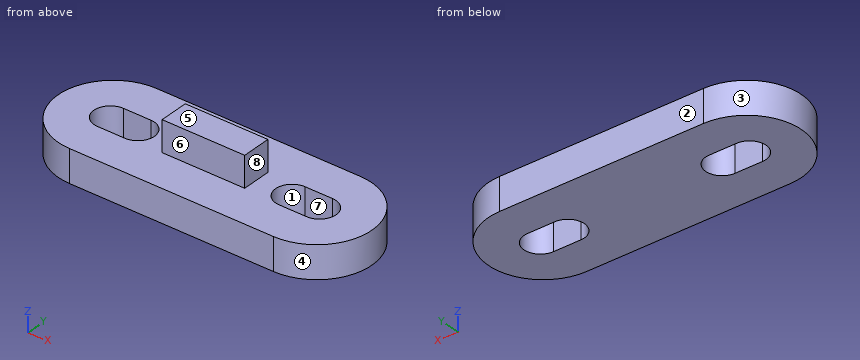
from build123d import *

# Parameters (mm, degrees)
BOSS_EXTRUDE2_DEPTH = 2.97
SKETCH5_W           = 7.5
SKETCH5_H           = 2.65
BOSS_EXTRUDE3_DEPTH = 2.8


with BuildPart() as part:
    # Sketch3 → Boss-Extrude2 (new body)
    with BuildSketch(Plane.XY):
        with BuildLine():
            Line((-9.25, 5), (9.25, 5))
            ThreePointArc((9.25, 5), (14.25, 0), (9.25, -5))
            Line((9.25, -5), (-9.25, -5))
            ThreePointArc((-9.25, -5), (-14.25, 0), (-9.25, 5))
        make_face()
        with BuildLine():
            Line((-9.5, 1.5), (-7, 1.5))
            ThreePointArc((-7, 1.5), (-5.5, 0), (-7, -1.5))
            Line((-7, -1.5), (-9.5, -1.5))
            ThreePointArc((-9.5, -1.5), (-11, 0), (-9.5, 1.5))
        make_face(mode=Mode.SUBTRACT)
        with BuildLine():
            Line((9.5, -1.5), (7, -1.5))
            ThreePointArc((7, -1.5), (5.5, 0), (7, 1.5))
            Line((7, 1.5), (9.5, 1.5))
            ThreePointArc((9.5, 1.5), (11, 0), (9.5, -1.5))
        make_face(mode=Mode.SUBTRACT)
    extrude(amount=BOSS_EXTRUDE2_DEPTH)

    # Sketch5 → Boss-Extrude3 (add)
    with BuildSketch(Plane.XY.offset(2.97)):
        Rectangle(SKETCH5_W, SKETCH5_H)
    extrude(amount=BOSS_EXTRUDE3_DEPTH)


solid = part.part
Check sheet for the modelled part. Datum: model origin and axes. Units: mm. Face numbers are marked on the shaded views. A direction names the side the tool comes from. Round coordinates to 2 decimals unless told otherwise and drop trailing zeros. Order: outer loops, then holes, each group sorted by start corner. A loop starts at its lowest first (then second) coordinate and runs counter-clockwise, first axis right, second up.
Q1. Draft check along Y on the marked faces 1, 2 and 3. Enter one of: pulls with the +Y half, pulls with the -Y half, needs draft (parallel to the pull), parting line crosses it, or undercut.
Filled sheet:
face 1: undercut
face 2: pulls with the +Y half
face 3: parting line crosses it
Q2. Cross-section at B-B, the plane x = -6.25. Enter the section's corners in (y, z).
Filled sheet:
outline: (-5, 0) - (-1.3, 0) - (-1.3, 2.97) - (-5, 2.97) - close; (1.3, 0) - (5, 0) - (5, 2.97) - (1.3, 2.97) - close
Q3. Scan lines: L1, parallel to X at y = 0.25, z = 1.95; L2, parallel to Z at x = -11, y = 4.5; L3, parallel to X at y = 0.5, z = 3.65. Record each from-to range of solid material in increasing order.
Filled sheet:
L1: x = -14.24 to -10.98, -5.52 to 5.52, 10.98 to 14.24
L2: z = 0 to 2.97
L3: x = -3.75 to 3.75
Q4. Cross-section at D-D, the plane z = 5.1. Enter the section's corners in (x, y) (3 decimals).
Filled sheet:
outline: (-3.75, -1.325) - (3.75, -1.325) - (3.75, 1.325) - (-3.75, 1.325) - close
Q5. Depth check by flat-ended pin: P1, Ø3, axis at x = 0.5, z = 4.5, coming from the +Y side (3 decimals); P2, Ø0.8, axis at y = 0.5, z = 4, coming from the -X side; P3, Ø2, axis at x = -1.5, z = 4.5, coming from the -Y side (3 decimals). Enter the tip coordinate at first touch or a pass-through.
Filled sheet:
P1: stops at y = 1.325
P2: stops at x = -3.75
P3: stops at y = -1.325
Q6. Cross-section at A-A, the plane y = 1. Enter the section's corners in (x, z), plus the area to 3 significant figures.
Filled sheet:
outline: (-14.15, 0) - (-10.62, 0) - (-10.62, 2.97) - (-14.15, 2.97) - close; (-5.88, 0) - (5.88, 0) - (5.88, 2.97) - (3.75, 2.97) - (3.75, 5.77) - (-3.75, 5.77) - (-3.75, 2.97) - (-5.88, 2.97) - close; (10.62, 0) - (14.15, 0) - (14.15, 2.97) - (10.62, 2.97) - close
area: 76.9 mm2
Q7. Cross-section at C-C, the plane x = 3.5. Enter the section's corners in (y, z) (3 decimals).
Filled sheet:
outline: (-5, 0) - (5, 0) - (5, 2.97) - (1.325, 2.97) - (1.325, 5.77) - (-1.325, 5.77) - (-1.325, 2.97) - (-5, 2.97) - close
Q8. Set-up check for the marked faces 4, 5, 6, 7 and 8: record each of +Z, -Z, +X, -X, +Y, -Y from which the full face is reachable in a straight line by a thin tool's end or side.
Filled sheet:
face 4: +Z, -Z, +X
face 5: +Z, +X, -X, +Y, -Y
face 6: +Z, +X, -X, -Y
face 7: +Z, -Z
face 8: +Z, +X, +Y, -Y
